from build123d import *

# Parameters (mm, degrees)
SKETCH1_W           = 200
SKETCH1_H           = 2
BOSS_EXTRUDE1_DEPTH = 60
SKETCH2_R           = 37
BOSS_EXTRUDE2_DEPTH = 5
FILLET1_R           = 2
FILLET2_R           = 3
SKETCH4_W           = 120
SKETCH4_H           = 2
CUT_EXTRUDE1_DEPTH  = 209.865985742


with BuildPart() as part:
    # Sketch1 → Boss-Extrude1 (new, symmetric)
    with BuildSketch(Plane.XY):
        with Locations((0, 1)):
            Rectangle(SKETCH1_W, SKETCH1_H)
    extrude(amount=BOSS_EXTRUDE1_DEPTH, both=True)

    # Sketch2 → Boss-Extrude2 (add)
    with BuildSketch(Plane.XZ):
        with Locations(Location((0, 0, 0), (0, 0, 270))):
            Circle(SKETCH2_R)
    extrude(amount=BOSS_EXTRUDE2_DEPTH)

    # Fillet1
    fillet1_edges = [part.edges().sort_by_distance(p)[0] for p in [
        (0, -5, 37),
    ]]
    fillet(fillet1_edges, radius=FILLET1_R)

    # Fillet2
    fillet2_edges = [part.edges().sort_by_distance(p)[0] for p in [
        (0, 0, 37),
    ]]
    fillet(fillet2_edges, radius=FILLET2_R - 0.0001)  # a hair under: the kernel refuses the full size

    # Sketch4 → Cut-Extrude1 (cut, through all)
    with BuildSketch(Plane.ZY.offset(100)):
        with Locations((0, 1)):
            Rectangle(SKETCH4_W, SKETCH4_H)
    extrude(amount=-CUT_EXTRUDE1_DEPTH, mode=Mode.SUBTRACT)


solid = part.part
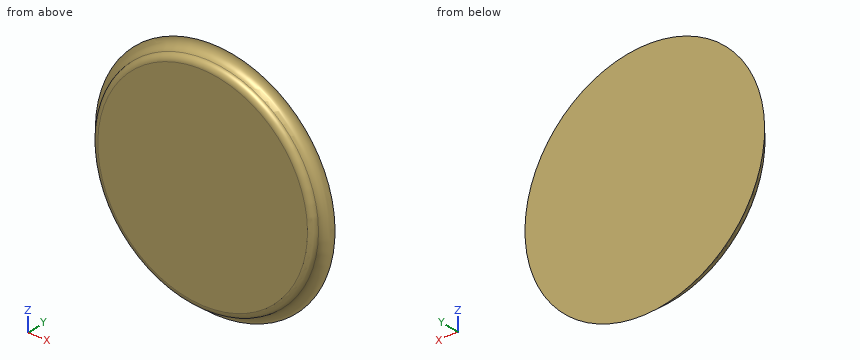
Source: CAD feature listing. Evaluate the final solid. Frame: model axes, mm. Give positions to 0.01 mm unless a question says otherwise; leave off trailing zeros. Write each loop counter-clockwise with the first axis right and the second up, starting at its lowest first coordinate (ties: lowest second). Pieces come first, ordered by that corner, then holes. Notation, with made-up numbers: M 63,68.25 L 105,68.25 A27 ccw 105,91.25 Z; hole C 44.5,73 d1. An arc over 180 degrees is marked long. Answer as a JSON object with one key per item and string values.
Q1. Cut plane C-C, the plane y = -1.1. Return the cut outline in (x, z).
Geometry check:
{"outline": "C 0,0 d75.36"}
Q2. Ray query, line 1 along X through (y, z) = (-3.15, -12); line 2 along X through (y, z) = (-2.4, -34); line 3 along Z through (x, y) = (20.5, -4.15). Return the intervals inside material, ascending.
Geometry check:
{"line 1": "x = -34.99 to 34.99", "line 2": "x = -14.75 to 14.75", "line 3": "z = -30.36 to 30.36"}
Q3. Contact query for flat-ended pins moving along their axis: P1, Ø2, axis at x = -24, z = -22.5, coming from the +Y side; P2, Ø3, axis at y = -3, z = 8.5, coming from the +X side. Output: stop coordinate, or through.
Geometry check:
{"P1": "stops at y = 0", "P2": "stops at x = 36.49"}
